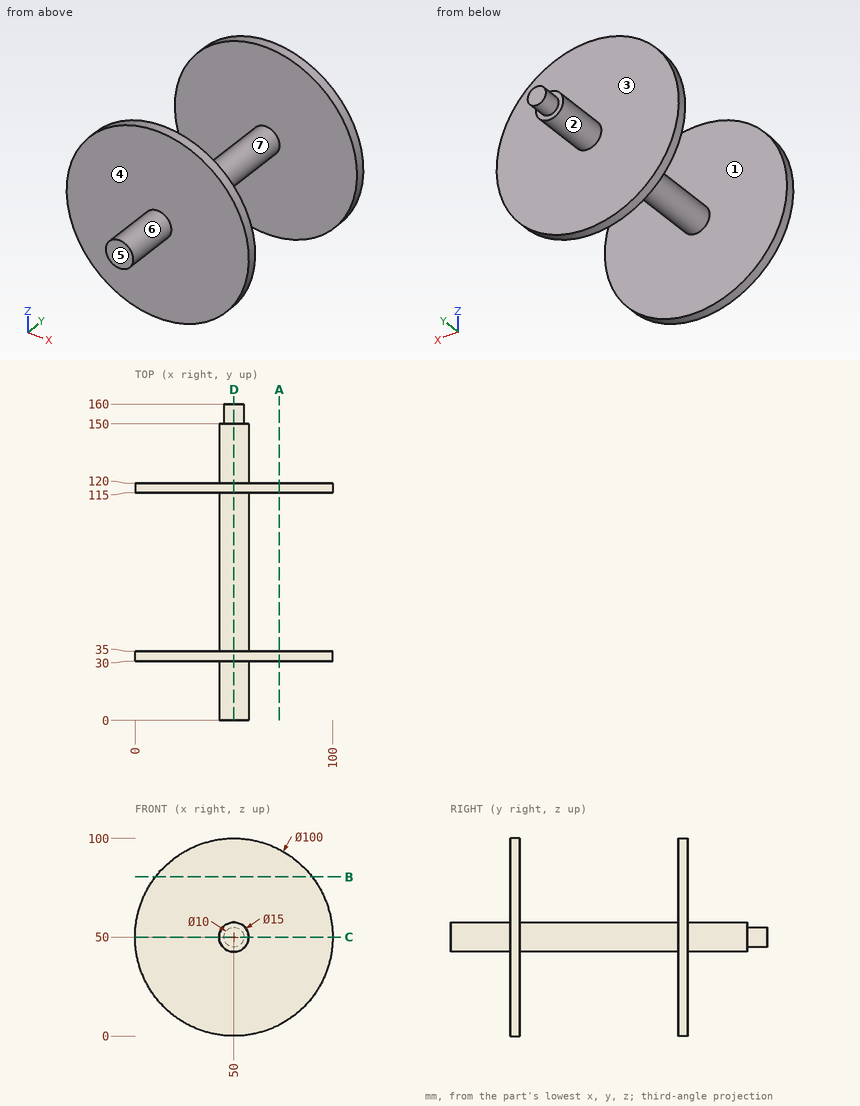
Verification items for this drawing (mm, ordinates from the low corner). A direction names the side the tool comes from. Give positions to 0.01 mm unless a question says otherwise; leave off trailing zeros. Loops run counter-clockwise (first coordinate to the right, second up) from the corner with the lowest first, then second, coordinate; pieces in that order, holes last. Notation, with made-up numbers: M -39,39.25 L -8,39.25 A16 cw -8,46.25 Z; hole C -25.75,79.25 d8. An arc over 180 degrees is marked long. Answer in a Markdown table with one row per item.
1) Depth check by flat-ended pin: pin 1 (1 mm diameter, centred on x = 73.5, z = 22.5, fed in from +Y); pin 2 (8 mm diameter, centred on x = 17, z = 30.5, fed in from -Y); pin 3 (1.5 mm diameter, centred on x = 51, y = 125.5, fed in from -Z). Enter the tip coordinate at first touch or a pass-through.
Solutions:
| item | result |
|---|---|
| pin 1 | stops at y = 120 |
| pin 2 | stops at y = 30 |
| pin 3 | stops at z = 42.5 |
2) Cross-section at B-B (z = 80.5). Enter the section's corners in (x, y), plus the area to 3 significant figures.
Solutions:
| item | result |
|---|---|
| outline | M 10.38,30 L 89.62,30 L 89.62,35 L 10.38,35 Z; M 10.38,115 L 89.62,115 L 89.62,120 L 10.38,120 Z |
| area | 792 mm^2 |
3) Tool access check on the marked faces 5, 6 and 7. Record the directions out of +Z, -Z, +X, -X, +Y, -Y that give a thin tool (end or side, any length) a straight path to the whole face; none if there is none.
Solutions:
| item | result |
|---|---|
| face 5 | +Z, -Z, +X, -X, -Y |
| face 6 | -Y |
| face 7 | none |
4) Cross-section at A-A (x = 73). Enter the section's corners in (y, z), plus the area to 3 significant figures.
Solutions:
| item | result |
|---|---|
| outline | M 30,5.6 L 35,5.6 L 35,94.4 L 30,94.4 Z; M 115,5.6 L 120,5.6 L 120,94.4 L 115,94.4 Z |
| area | 888 mm^2 |
5) Cross-section at C-C (z = 50). Enter the section's corners in (x, y), plus the area to 3 significant figures.
Solutions:
| item | result |
|---|---|
| outline | M 0,30 L 42.5,30 L 42.5,0 L 57.5,0 L 57.5,30 L 100,30 L 100,35 L 57.5,35 L 57.5,115 L 100,115 L 100,120 L 57.5,120 L 57.5,150 L 55,150 L 55,160 L 45,160 L 45,150 L 42.5,150 L 42.5,120 L 0,120 L 0,115 L 42.5,115 L 42.5,35 L 0,35 Z |
| area | 3,200 mm^2 |
6) Mould release check, pull along Y, two halves, no side actions. Record for the marked faces 1, 2, 3 and 4: released by +Y, released by -Y, zero draft, split by the parting line, or undercut.
Solutions:
| item | result |
|---|---|
| face 1 | undercut |
| face 2 | zero draft |
| face 3 | released by +Y |
| face 4 | released by -Y |
7) Thickness scan on line 1 (Y direction, x = 14, z = 24); line 2 (X direction, y = 118.5, z = 55); line 3 (X direction, y = 117, z = 74). Record the ranges inside material, lowest first.
Solutions:
| item | result |
|---|---|
| line 1 | y = 30 to 35, 115 to 120 |
| line 2 | x = 0.25 to 99.75 |
| line 3 | x = 6.14 to 93.86 |
8) Cross-section at D-D (x = 50). Enter the section's corners in (y, z).
Solutions:
| item | result |
|---|---|
| outline | M 0,42.5 L 30,42.5 L 30,0 L 35,0 L 35,42.5 L 115,42.5 L 115,0 L 120,0 L 120,42.5 L 150,42.5 L 150,45 L 160,45 L 160,55 L 150,55 L 150,57.5 L 120,57.5 L 120,100 L 115,100 L 115,57.5 L 35,57.5 L 35,100 L 30,100 L 30,57.5 L 0,57.5 Z |
